The model under review builds one solid part; all positions refer to its coordinate system, in mm. A direction names the side the tool comes from. Coordinates: 2 decimals unless noted, no trailing zeros. Write each loop counter-clockwise with the first axis right and the second up, starting at its lowest first coordinate (ties: lowest second). Pieces come first, ordered by that corner, then holes. Notation, with made-up numbers: (42, 38.25) - (69, 38.25) arc R20 ccw to (69, 43.25) - close; hole circle Ø8 at (34, 19.5). An arc over 180 degrees is marked (long way). Answer as CSV lines item,"result". Start each with the question number.
Autodesk Inventor part; units mm, degrees
ref_plane "YZ Plane" through (0, 0, 0) normal (1, 0, 0) x (0, 1, 0)
ref_plane "XZ Plane" through (0, 0, 0) normal (0, 1, 0) x (-1, 0, 0)
ref_plane "XY Plane" through (0, 0, 0) normal (0, 0, 1) x (1, 0, 0)
sketch "Sketch1" plane through (0, 0, 0) normal (0, 0, 1) x (1, 0, 0)
  line L0 (0, 0) -> (88.9, 0)
  line L1 (88.9, 0) -> (88.9, 25.4)
  line L2 (88.9, 25.4) -> (0, 25.4)
  line L3 (0, 25.4) -> (0, 0)
  dimension "d0" = 25.4
  dimension "d1" = 88.9
extrude "Extrusion1" add sketch "Sketch1" along normal blind 73.279
sketch "Sketch2" plane through (0, 25.4, 0) normal (0, 1, 0) x (1, 0, 0)
  line L0 (0, -44.4754) -> (0, -28.575)
  line L1 (0, -28.575) -> (12.7, -28.575)
  line L2 (0, -44.4754) -> (12.7, -44.4754)
  arc A0 (12.7, -44.4754) -> (12.7, -28.575) centre (12.7, -36.5252) ccw
  line L3 (88.9, 0) -> (0, 0)
  line L4 (0, 0) -> (0, -73.279)
  dimension "d5" = 36.5252
  dimension "d6" = 7.9502
  dimension "d7" = 12.7
  dimension "d8" = 0
  dimension "d9" = 12.7
  dimension "d10" = 12.7
extrude "Extrusion2" cut sketch "Sketch2" against normal blind 73.279
sketch "Sketch3" plane through (0, 25.4, 0) normal (0, 1, 0) x (1, 0, 0)
  line L0 (0, -73.279) -> (88.9, -73.279)
  line L1 (63.5, -73.279) -> (88.9, -55.753)
  line L2 (88.9, 0) -> (88.9, -73.279)
  line L3 (88.9, -73.279) -> (63.5, -73.279)
  line L4 (88.9, -73.279) -> (88.9, -55.753)
  line L5 (63.5, 0) -> (88.9, 0)
  line L6 (88.9, 0) -> (0, 0)
  line L7 (88.9, -17.526) -> (63.5, 0)
  line L8 (88.9, -17.526) -> (88.9, 0)
  line L9 (0, -44.4754) -> (0, -73.279)
  line L10 (0, 0) -> (0, -28.575)
  dimension "d13" = 17.526
  dimension "d14" = 17.526
  dimension "d15" = 63.5
  dimension "d16" = 63.5
extrude "Extrusion3" cut sketch "Sketch3" against normal blind 73.279
sketch "Sketch4" plane through (88.9, 0, 55.753) normal (1, 0, 0) x (0, 0, -1)
  line L0 (0, 25.4) -> (0, 0)
  line L1 (55.753, 25.4) -> (27.178, 25.4)
  line L2 (6.2992, 0) -> (32.0802, 0)
  line L3 (32.0802, 0) -> (32.0802, 25.4)
  line L4 (32.0802, 25.4) -> (6.2992, 25.4)
  line L5 (6.2992, 25.4) -> (6.2992, 0)
  line L6 (-17.526, 0) -> (-17.526, 25.4)
  point P0 (55.753, 0)
  dimension "d19" = 25.781
  dimension "d20" = 23.8252
extrude "Extrusion4" cut sketch "Sketch4" against normal blind 25.4
chamfer "Chamfer1" distance 1.524 angle 45 6 edges at (31.75, 25.4, 73.279) (76.2, 25.4, 64.516) (88.9, 25.4, 52.6034) (88.9, 25.4, 20.5994) (76.2, 25.4, 8.763) (31.75, 25.4, 0)
sketch "Sketch5" plane through (0, 25.4, 28.575) normal (0, 1, 0) x (1, 0, 0)
  line L0 (0, 27.051) -> (0, 0)
  line L1 (63.5, 28.575) -> (0, 28.575)
  point P0 (26.9748, -7.9502)
  dimension "d26" = 26.9748
  dimension "d27" = 36.5252
hole "Hole1" at (26.9748, 25.4, 36.5252) direction (0, -1, 0) diameter 6.477 depth 14.2748 tip angle 118
sketch "Sketch6" plane through (63.5, 0, 55.753) normal (1, 0, 0) x (0, 0, -1)
  line L0 (6.2992, 25.4) -> (32.0802, 25.4)
  line L1 (6.2992, 0) -> (6.2992, 23.876)
  point P0 (55.753, 0)
  point P1 (19.1897, 12.7)
  dimension "d35" = 12.7
  dimension "d36" = 12.8905
hole "Hole2" at (63.5, 12.7, 36.5633) direction (-1, 0, 0) diameter 9.525 depth 19.05 tip angle 118
properties part number "7.2 Q6"
(1) Add section C-C on y = 22.5. Give the boundary of the cut face in (x, z) (1 decimal).
(2) The part is to be moulded in two halves that separate along Z. For faces 1 (the flat face through (6, 13, 28.575)), 2 (the flat face through (76.4, 12.1, 8.9)), 3 (the flat face through (35, 25.4, 36)), say which applies: released by +Z, released by -Z, zero draft, split by the parting line, or undercut.
(3) For faces 4 (the cylindrical face through (30.136, 18.163, 35.823)), 5 (the flat face through (6, 13, 44.475)), 6 (the flat face through (76, 13, 23.673)), 7 (the flat face through (31, 12, 73.279)), list the 3-axis set-ups (+Z, -Z, +X, -X, +Y, -Y) from which the entire face can be reached by the end or side of a thin tool; tool diameter is ignored.
(4) Add section D-D on z = 8.5. Give the boundary of the cut face in (x, y).
(5) For pin 1 (7.5 mm diameter, centred on x = 70.5, y = 13.5, fed in from -Z); pin 2 (1 mm diameter, centred on x = 68.5, y = 9.5, fed in from -Z) (3 decimals); pin 3 (12.5 mm diameter, centred on y = 12.7, z = 36.56, fed in from -X), all flat-tipped, find the tip position at first contact; note any pin that passes through.
(6) Wall thickness on line 1 (Z direction, x = 10, y = 15.25) (3 decimals); line 2 (Z direction, x = 55.25, y = 12.7); line 3 (X direction, y = 22.75, z = 10): over which ranges is each line inside the solid? List them lowest first.
(7) Add section B-B on y = 3.25. Give the boundary of the cut face in (x, z) (3 decimals), then the cut area to 3 significant figures.
(8) Add section A-A on x = 66.5. Give the boundary of the cut face in (y, z), then the cut area to 3 significant figures.
Reported:
1,outline,"(0, 0) - (63.5, 0) - (88.9, 17.5) - (88.9, 23.7) - (63.5, 23.7) - (63.5, 49.5) - (88.9, 49.5) - (88.9, 55.8) - (63.5, 73.3) - (0, 73.3) - (0, 44.5) - (12.7, 44.5) arc R8 cw to (12.7, 28.6) - (0, 28.6) - close; hole circle Ø6.5 at (27, 36.5)"
2,face 1,"undercut"
2,face 2,"released by -Z"
2,face 3,"zero draft"
3,face 4,"+Y"
3,face 5,"-X, +Y, -Y"
3,face 6,"+X, +Y, -Y"
3,face 7,"+Z, +X, -X, +Y, -Y"
4,outline,"(0, 0) - (75.82, 0) - (75.82, 23.88) - (73.14, 25.4) - (0, 25.4) - close"
5,pin 1,"z = 2.24"
5,pin 2,"z = 3.105"
5,pin 3,"x = 17.57"
6,line 1,"0 to 28.575, 44.475 to 73.279"
6,line 2,"0 to 31.8, 41.33 to 73.28"
6,line 3,"0 to 77.99"
7,outline,"(0, 0) - (63.5, 0) - (88.9, 17.526) - (88.9, 23.673) - (63.5, 23.673) - (63.5, 49.454) - (88.9, 49.454) - (88.9, 55.753) - (63.5, 73.279) - (0, 73.279) - (0, 44.475) - (12.7, 44.475) arc R7.95 cw to (12.7, 28.575) - (0, 28.575) - close"
7,area,"5,110 mm²"
8,outline,"(0, 2.07) - (23.88, 2.07) - (25.4, 3.92) - (25.4, 23.67) - (0, 23.67) - close; (0, 49.45) - (25.4, 49.45) - (25.4, 69.36) - (23.88, 71.21) - (0, 71.21) - close"
8,area,"1,100 mm²"
